from build123d import *

# Parameters (mm, degrees)
SKETCH017_W     = 16
SKETCH017_H     = 15.8
PAD010_DEPTH    = 28.8
POCKET007_DEPTH = 16
PAD137_DEPTH    = 15.8


with BuildPart() as part:
    # Sketch017 (on Face68 of Binder006) → Pad010 (new body)
    with BuildSketch(Plane.XY.offset(-28.8)):
        with Locations((-8, 127.9)):
            Rectangle(SKETCH017_W, SKETCH017_H)
    extrude(amount=PAD010_DEPTH)

    # Sketch018 (on Face3 of Pad010) → Pocket007 (cut)
    with BuildSketch(Plane.XZ.offset(-120)):
        Polygon((0, 0), (-16, -9.6), (-16, 0), align=None)
    extrude(amount=-POCKET007_DEPTH, mode=Mode.SUBTRACT)

    # Sketch141 (on Face6 of Pocket007) → Pad137 (join)
    with BuildSketch(Plane.XZ.offset(-120)):
        Polygon((0, 0), (-3.2, 0), (-16, -7.68), (-16, -10.88), (-3.2, -3.2), (0, -3.2), align=None)
    extrude(amount=-PAD137_DEPTH)


solid = part.part
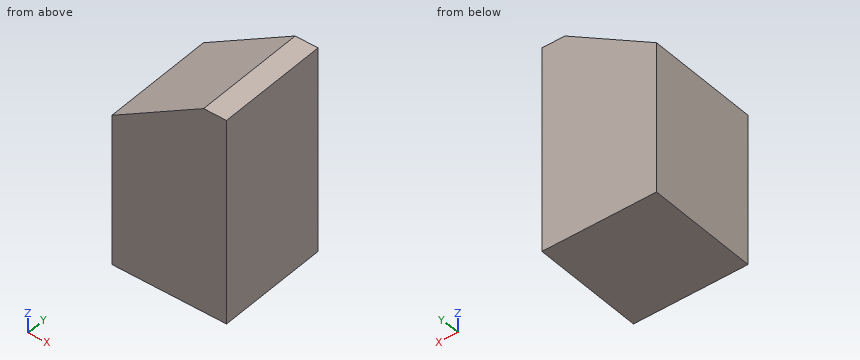
Geometry: final body of the model. Coordinates: model frame, mm. Give positions to 0.01 mm unless a question says otherwise; leave off trailing zeros. Write each loop counter-clockwise with the first axis right and the second up, starting at its lowest first coordinate (ties: lowest second). Pieces come first, ordered by that corner, then holes. Notation, with made-up numbers: (14.5, 84.25) - (35.5, 84.25) arc R31 ccw to (35.5, 108.25) - close; hole circle Ø4 at (82.5, -19). An arc over 180 degrees is marked (long way). Return JSON: item names as keys, results as strings. Group by question number.
1) Section B-B on x = -8.5. Return the cut outline in (y, z), plus the area to 3 significant figures.
2) First-contact query: P1, Ø2, axis at x = -4.5, y = 124, coming from the +Z side; P2, Ø1, axis at x = -5.5, y = 129.5, coming from the +Z side; P3, Ø2, axis at x = -10.5, y = 124.5, coming from the +Z side. Flat tips, straight axial feed; report the tip coordinate or a pass-through.
3) Section C-C on z = -5.25. Return the cut outline in (x, y).
4) Line query: line 1 (X direction, y = 131.5, z = -6); line 2 (Z direction, x = -7.25, y = 120.5); line 3 (X direction, y = 127, z = -6.75). Output: solid intervals per line, ascending.
5) Section A-A on y = 134. Return the cut outline in (x, z), plus the area to 3 significant figures.
Filled in:
{
 "1": {"outline": "(120, -28.8) - (135.8, -28.8) - (135.8, -3.18) - (120, -3.18) - close", "area": "405 mm^2"},
 "2": {"P1": "stops at z = -0.18", "P2": "stops at z = -1.08", "P3": "stops at z = -3.78"},
 "3": {"outline": "(-11.95, 120) - (0, 120) - (0, 135.8) - (-11.95, 135.8) - close"},
 "4": {"line 1": "x = -13.2 to 0", "line 2": "z = -28.8 to -2.43", "line 3": "x = -14.45 to 0"},
 "5": {"outline": "(-16, -28.8) - (0, -28.8) - (0, 0) - (-3.2, 0) - (-16, -7.68) - close", "area": "412 mm^2"}
}
